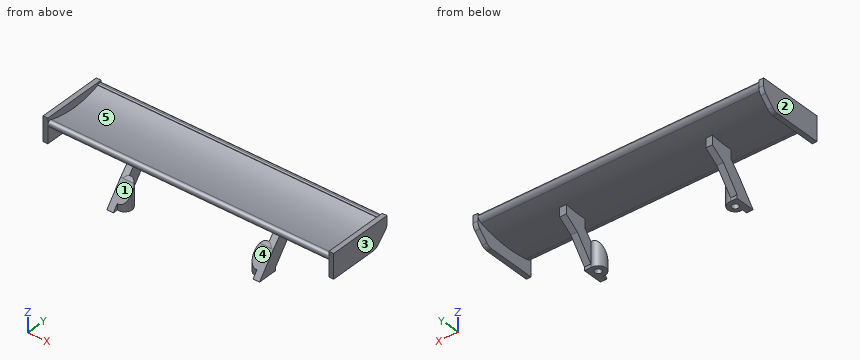
from build123d import *

# Parameters (mm, degrees)
F4_W      = 15
F4_H      = 5.6
F5_DEPTH  = 1.1
F6_SIZE   = 3.1
F7_W      = 15
F7_H      = 5.6
F8_DEPTH  = 1.1
F9_SIZE   = 3.1
F11_DEPTH = 32.2
F12_R     = 0.25
F13_R     = 2
F15_DEPTH = 1.5
F17_DEPTH = 1.5
F18_R     = 1.7
F19_DEPTH = 6.8
F22_W     = 36
F22_H     = 4
F24_R     = 0.75
F25_DEPTH = 2.5


with BuildPart() as f5:
    # F4 (on offset) → F5 (new body)
    with BuildSketch(Plane.YZ.offset(33.3)):
        with Locations((7.5, 2.8)):
            Rectangle(F4_W, F4_H)
    extrude(amount=-F5_DEPTH)

    # F6
    f6_edges = [f5.edges().sort_by_distance(p)[0] for p in [
        (32.75, 15, 0),
    ]]
    chamfer(f6_edges, length=F6_SIZE)



with BuildPart() as f8:
    # F7 (on offset) → F8 (new body)
    with BuildSketch(Plane.YZ.offset(-33.3)):
        with Locations((7.5, 2.8)):
            Rectangle(F7_W, F7_H)
    extrude(amount=F8_DEPTH)

    # F9
    f9_edges = [f8.edges().sort_by_distance(p)[0] for p in [
        (-32.75, 15, 0),
    ]]
    chamfer(f9_edges, length=F9_SIZE)


with BuildPart() as f5_1:
    add(f5.part)

    add(f8.part)  # F11 merges F8
    # F10 (on Right) → F11 (join, symmetric)
    with BuildSketch(Plane.YZ):
        with BuildLine():
            ThreePointArc((14.1, 4.9799904701), (7.5241974898, 3.7896224533), (0.9153141097, 4.7799835677))
            ThreePointArc((0.9153141097, 4.7799835677), (0.075756099, 4.4131641565), (0.3380033304, 3.5353028215))
            ThreePointArc((0.3380033304, 3.5353028215), (0.8766544844, 3.272139492), (1.4572901418, 3.1229341403))
            ThreePointArc((1.4572901418, 3.1229341403), (7.8107981998, 2.7603942388), (14.0573066811, 3.9767953297))
            ThreePointArc((14.0573066811, 3.9767953297), (14.7402257131, 4.4876667413), (15, 5.3))
            Line((15, 5.3), (14.1, 5.3))
            Line((14.1, 5.3), (14.1, 4.9799904701))
        make_face()
    extrude(amount=F11_DEPTH, both=True)

    # F12
    f12_edges = [f5_1.edges().sort_by_distance(p)[0] for p in [
        (0, 14.1, 5.3),
        (0, 15, 5.3),
    ]]
    fillet(f12_edges, radius=F12_R)

    # F13
    f13_edges = [f5_1.edges().sort_by_distance(p)[0] for p in [
        (32.75, 11.9, 0),
        (32.75, 15, 3.1),
        (-32.75, 15, 3.1),
        (-32.75, 11.9, 0),
    ]]
    fillet(f13_edges, radius=F13_R)

    # F14 (on offset) → F15 (join)
    with BuildSketch(Plane.YZ.offset(-16)):
        with BuildLine():
            ThreePointArc((10, 3.0037642772), (7.4076873546, 2.736270416), (4.8016114163, 2.7338166819))
            Line((4.8016114163, 2.7338166819), (4.8016114163, 0.7338166819))
            Line((4.8016114163, 0.7338166819), (2.4397989119, -1.9831378069))
            Line((2.4397989119, -1.9831378069), (-1.4298789153, -6.9614928532))
            Line((-1.4298789153, -6.9614928532), (3.0701210847, -6.9614928532))
            Line((3.0701210847, -6.9614928532), (3.0701210847, -6.1614928532))
            Line((3.0701210847, -6.1614928532), (6.8872222317, -1.2758261809))
            Line((6.8872222317, -1.2758261809), (10, 0.9037642772))
            Line((10, 0.9037642772), (10, 3.0037642772))
        make_face()
    extrude(amount=-F15_DEPTH)

    # F16 (on offset) → F17 (join)
    with BuildSketch(Plane.YZ.offset(16)):
        with BuildLine():
            Line((2.4397989119, -1.9831378069), (-1.4298789153, -6.9614928532))
            Line((-1.4298789153, -6.9614928532), (3.0701210847, -6.9614928532))
            Line((3.0701210847, -6.9614928532), (3.0701210847, -6.1614928532))
            Line((3.0701210847, -6.1614928532), (6.8872222317, -1.2758261809))
            Line((6.8872222317, -1.2758261809), (10, 0.9037642772))
            Line((10, 0.9037642772), (10, 3.0037642772))
            ThreePointArc((10, 3.0037642772), (7.4076873546, 2.736270416), (4.8016114163, 2.7338166819))
            Line((4.8016114163, 2.7338166819), (4.8016114163, 0.7338166819))
            Line((4.8016114163, 0.7338166819), (2.4397989119, -1.9831378069))
        make_face()
    extrude(amount=F17_DEPTH)

    # F18 (on face) → F19 (join)
    with BuildSketch(Plane(origin=(0, 0, -6.9614928532), x_dir=(1, 0, 0), z_dir=(0, 0, -1))):
        with BuildLine():
            Line((-16, -3.0434411378), (-16, 0.3031989684))
            ThreePointArc((-16, 0.3031989684), (-17.4, -1.3701210847), (-16, -3.0434411378))
        make_face()
        with BuildLine():
            ThreePointArc((-16, -3.0434411378), (-14.6091287885, -2.6739615657), (-14, -1.3701210847))
            ThreePointArc((-14, -1.3701210847), (-14.6091287885, -0.0662806036), (-16, 0.3031989684))
            Line((-16, 0.3031989684), (-16, -3.0434411378))
        make_face()
        with Locations((15.7, -1.3701210847)):
            Circle(F18_R)
    extrude(amount=-F19_DEPTH)

    # F23: sweep along a path in F20
    with BuildLine(Plane(origin=(-17.5, 0, 0), x_dir=(0, -1, 0), z_dir=(-1, 0, 0))) as f23_path:
        Line((-3.7519169699, -0.4737186464), (-2.4397989119, -1.9831378069))
        Line((-2.4397989119, -1.9831378069), (1.4298789153, -6.9614928532))
    # F22 (on face) → F23 (sweep, cut)
    with BuildSketch(Plane(origin=(0, -3.9117899018, -5.0321591222), x_dir=(1, 0, 0), z_dir=(0, 0.6137341658, 0.7895127445))):
        with Locations((0, 1.1435983825)):
            Rectangle(F22_W, F22_H)
    sweep(path=f23_path.line, transition=Transition.RIGHT, mode=Mode.SUBTRACT)

    # F24 (on face) → F25 (cut)
    with BuildSketch(Plane(origin=(0, 0, -6.9614928532), x_dir=(1, 0, 0), z_dir=(0, 0, -1))):
        with Locations((-15.7, -1.3701210847)):
            Circle(F24_R)
        with Locations((15.7, -1.3701210847)):
            Circle(F24_R)
    extrude(amount=-F25_DEPTH, mode=Mode.SUBTRACT)


solid = f5_1.part
Could you check a few things on this model? Use its own coordinates, in mm. Face numbers are marked on the shaded views. A direction names the side the tool comes from. Give positions to 0.01 mm unless a question says otherwise; leave off trailing zeros. Order: outer loops, then holes, each group sorted by start corner. A loop starts at its lowest first (then second) coordinate and runs counter-clockwise, first axis right, second up. Notation, with made-up numbers: (-12.5, 72) - (-3.5, 72) arc R20 cw to (-3.5, 100) - close; hole circle Ø4 at (87.5, 24.5). An arc over 180 degrees is marked (long way). One line per item, written item: value. Start each with the question number.
1. For the marked faces 1 and 2, which set-ups out of +Z, -Z, +X, -X, +Y, -Y let a thin tool reach every point of the face, with its end or its side?
2. Thinking about a two-plate mould opening in Z: for the marked faces 3, 4 and 5, which applies, +Z half, -Z half, draft (parallel to the pull), parting line (faces both ways), or undercut?
3. If I drill on probe 1 along Y at (x, z) = (15.7, -5.6); probe 2 along X at (y, z) = (4.5, 1.75); probe 3 along X at (y, z) = (5.75, -1), over which ranges is the centre line in solid material (lowest first)?
4. Imagine slicing it at B-B on x = -19.5. List the corners of the cut face in (y, z) for me, plus the area to 3 significant figures.
5. Imagine slicing it at A-A on y = 9.25. List the corners of the cut face in (x, z) for me.
6. For P1, Ø0.9, axis at x = 16.5, z = -7, coming from the +Y side; P2, Ø2, axis at x = -15.7, y = 1.37, coming from the +Z side; P3, Ø6, axis at x = -26, y = 6.5, coming from the +Z side, each with a flat end and sliding along its axis, tell me the tip position at first contact or that it passes through.
Values:
1. face 1: +X, -X, -Y
1. face 2: +Z, -Z, -X, +Y, -Y
2. face 3: draft
2. face 4: undercut
2. face 5: +Z half
3. probe 1: -0.33 to 0.62, 2.12 to 3.07
3. probe 2: -33.3 to -32.2, 32.2 to 33.3
3. probe 3: -17.5 to -16, 16 to 17.5
4. outline: (0.34, 3.54) arc R2.96 ccw to (1.46, 3.12) arc R25.59 ccw to (14.06, 3.98) arc R1.4 ccw to (14.97, 5) arc R0.25 ccw to (14.72, 5.3) - (14.35, 5.3) arc R0.25 ccw to (14.1, 5.05) - (14.1, 4.98) arc R20.48 cw to (0.92, 4.78) arc R0.69 ccw to start
4. area: 16.7 mm²
5. outline: (-33.3, 0) - (-32.2, 0) - (-32.2, 2.9) - (-17.5, 2.9) - (-17.5, 0.38) - (-16, 0.38) - (-16, 2.9) - (16, 2.9) - (16, 0.38) - (17.5, 0.38) - (17.5, 2.9) - (32.2, 2.9) - (32.2, 0) - (33.3, 0) - (33.3, 5.6) - (32.2, 5.6) - (32.2, 3.89) - (-32.2, 3.89) - (-32.2, 5.6) - (-33.3, 5.6) - close
6. P1: y = 3.07
6. P2: z = 4.81
6. P3: z = 4.13
